Autodesk Inventor part; units mm, degrees
ref_plane "YZ Plane" through (0, 0, 0) normal (1, 0, 0) x (0, 1, 0)
ref_plane "XZ Plane" through (0, 0, 0) normal (0, 1, 0) x (-1, 0, 0)
ref_plane "XY Plane" through (0, 0, 0) normal (0, 0, 1) x (1, 0, 0)
sketch "Sketch1" plane through (0, 0, 0) normal (0, 1, 0) x (-1, 0, 0)
  line L0 (-100, -260) -> (100, -260)
  line L1 (100, -260) -> (100, 260)
  line L2 (100, 260) -> (-100, 260)
  line L3 (-100, 260) -> (-100, -260)
  line L4 (-100, -260) -> (100, 260) construction
  line L5 (100, -260) -> (-100, 260) construction
  point P0 (0, 0)
  dimension "d0" = 200
  dimension "d1" = 520
extrude "Extrusion1" add sketch "Sketch1" along normal blind 10
fillet "Fillet1" radius 25 4 edges at (-100, 5, -260) (-100, 5, 260) (100, 5, 260) (100, 5, -260)
sketch "Sketch3" plane through (0, 10, 0) normal (0, 1, 0) x (1, 0, 0)
  line L0 (-75, -260) -> (75, -260)
  line L1 (-100, 235) -> (-100, -235)
  point P0 (0, 0)
  point P1 (-10, -245)
  point P2 (55, -245)
  dimension "d20" = 15
  dimension "d21" = 90
  dimension "d22" = 65
  dimension "d23" = 15
hole "Hole2" at (-10, 10, 245) at (55, 10, 245) direction (0, -1, 0) diameter 6.647 end through all
mirror "Mirror1" about plane through (0, 0, 0) normal (0, 0, 1) of "Hole2"
sketch "Sketch4" plane through (0, 10, 0) normal (0, 1, 0) x (1, 0, 0)
  line L0 (75, 260) -> (-75, 260)
  line L1 (100, -235) -> (100, 235)
  point P0 (0, 0)
  point P1 (-45, 30)
  point P2 (85, 30)
  dimension "d31" = 230
  dimension "d32" = 145
  dimension "d33" = 230
  dimension "d34" = 15
hole "Hole3" at (-45, 10, -30) at (85, 10, -30) direction (0, -1, 0) diameter 6.647 end through all
sketch "Sketch12" plane through (0, 0, 0) normal (0, -1, 0) x (1, 0, 0)
  line L0 (0, 0) -> (-38.9736, 0) construction
  line L1 (-100, -235) -> (-100, 235) construction
  point P0 (-74, 10)
  point P1 (-74, -10)
  point P2 (-58, 0)
  dimension "d109" = 10
  dimension "d110" = 26
  dimension "d111" = 16
hole "Hole8" at (-74, 0, 10) at (-74, 0, -10) at (-58, 0, 0) direction (0, 1, 0) diameter 3.242 end through all
sketch "Sketch8" plane through (0, 10, 0) normal (0, 1, 0) x (1, 0, 0)
  line L0 (-100, 235) -> (-100, -235)
  line L1 (-100, -125) -> (-75, -125)
  line L2 (-75, -125) -> (-75, -195)
  line L3 (-75, -195) -> (-100, -195)
  line L4 (-100, -195) -> (-100, -125)
  line L5 (-75, -260) -> (75, -260)
  point P0 (0, 0)
  dimension "d72" = 25
  dimension "d73" = 70
  dimension "d74" = 65
extrude "Extrusion2" cut sketch "Sketch8" against normal blind 10
fillet "Fillet2" radius 10 4 edges at (-100, 5, 125) (-75, 5, 125) (-100, 5, 195) (-75, 5, 195)
sketch "Sketch13" plane through (0, 10, 0) normal (0, 1, 0) x (1, 0, 0)
  line L0 (-100, 235) -> (-100, -115) construction
  line L1 (-100, 0) -> (0, 0) construction
  point P0 (-95, -43)
  point P1 (-95, 43)
  dimension "d119" = 86
  dimension "d120" = 5
hole "Hole9" at (-95, 10, 43) at (-95, 10, -43) direction (0, -1, 0) diameter 4.917 end through all
sketch "Sketch9" plane through (0, 10, 0) normal (0, 1, 0) x (1, 0, 0)
  line L0 (-90, 55) -> (-100, 55)
  line L1 (-100, 55) -> (-100, -55)
  line L2 (-100, -55) -> (-90, -55)
  line L3 (-90, -55) -> (-90, 55)
  line L4 (-100, 235) -> (-100, -115)
  line L5 (75, 260) -> (-75, 260)
  line L6 (0, 0) -> (-100, 0) construction
  dimension "d78" = 10
  dimension "d79" = 110
  dimension "d80" = 0
sketch "Sketch10" plane through (0, 10, 0) normal (0, 1, 0) x (1, 0, 0)
  line L0 (-30, 180) -> (-60, 180)
  line L1 (-60, 180) -> (-60, 110)
  line L2 (-60, 110) -> (-30, 110)
  line L3 (-30, 110) -> (-30, 180)
  line L4 (-100, 235) -> (-100, -115)
  line L5 (75, 260) -> (-75, 260)
  point P0 (0, 0)
  dimension "d85" = 30
  dimension "d86" = 70
  dimension "d87" = 40
  dimension "d88" = 80
sketch "Sketch11" plane through (0, 10, 0) normal (0, 1, 0) x (1, 0, 0)
  line L0 (-100, 235) -> (-100, -115)
  line L1 (-100, -205) -> (-100, -235)
  line L2 (75, 260) -> (-75, 260)
  line L3 (-75, -260) -> (75, -260)
  point P0 (0, 0)
  point P1 (-50, 220)
  point P2 (-50, 70)
  point P3 (-50, -80)
  point P4 (-50, -155)
  point P5 (-50, -230)
  dimension "d92" = 50
  dimension "d93" = 50
  dimension "d94" = 50
  dimension "d95" = 50
  dimension "d96" = 50
  dimension "d97" = 40
  dimension "d98" = 190
  dimension "d99" = 180
  dimension "d100" = 105
  dimension "d101" = 30
properties part number "Top_plate" material "Stainless Steel"
Geometry check sheet. Reference: the model listing, model coordinates, mm. A direction names the side the tool comes from. Round coordinates to 2 decimals unless told otherwise and drop trailing zeros. Use a Markdown table: item, result.
(1) Sectioned sample at A-A (y = 2.5). Give the number of separate pieces and of enclosed holes in the cut face, then the cut area to 3 significant figures.
Calculated:
| item | result |
|---|---|
| separate pieces | 1 |
| enclosed holes | 11 |
| area | 101,000 mm² |
(2) Set-up check for faces 4 (the flat face through (100, 5, 3)), 5 (the cylindrical face through (-96.99, 4.93, 122.15)): record each of +Z, -Z, +X, -X, +Y, -Y from which the full face is reachable in a straight line by a thin tool's end or side.
Calculated:
| item | result |
|---|---|
| face 4 | +Z, -Z, +X, +Y, -Y |
| face 5 | -X, +Y, -Y |
(3) Go/stop test with flat-tipped pins: P1, Ø3, axis at x = -58, z = 0, coming from the -Y side; P2, Ø5.5, axis at x = -87.5, y = 5, coming from the +Z side; P3, Ø12, axis at x = -52, z = 150.5, coming from the -Y side; P4, Ø2.5, axis at x = -87.5, y = 3, coming from the -Z side. Record where each tip stops, or that it passes through.
Calculated:
| item | result |
|---|---|
| P1 | through |
| P2 | z = 258.02 |
| P3 | y = 0 |
| P4 | z = -257.33 |
(4) Mould release check, pull along Z, two halves, no side actions. Record for faces 1 (the cylindrical face through (-77.85, 4.93, 191.99)), 2 (the cylindrical face through (92.871, 5.07, -252.482)), 3 (the cylindrical face through (92.482, 5.07, 252.871)): released by +Z, released by -Z, zero draft, split by the parting line, or undercut.
Calculated:
| item | result |
|---|---|
| face 1 | undercut |
| face 2 | released by -Z |
| face 3 | released by +Z |
(5) Scan lines: probe 1 along Z at (x, y) = (54.5, 2.25); probe 2 along X at (y, z) = (5, 0); probe 3 along X at (y, z) = (5, 245). Record each from-to range of solid material in increasing order.
Calculated:
| item | result |
|---|---|
| probe 1 | -260 to -248.29, -241.71 to 241.71, 248.29 to 260 |
| probe 2 | -100 to -59.62, -56.38 to 100 |
| probe 3 | -97.91 to -13.32, -6.68 to 51.68, 58.32 to 97.91 |
